Design review of the part built by this model. Coordinates are the model's own, in mm. A direction names the side the tool comes from. Give positions to 0.01 mm unless a question says otherwise; leave off trailing zeros. Loops run counter-clockwise (first coordinate to the right, second up) from the corner with the lowest first, then second, coordinate; pieces in that order, holes last. Notation, with made-up numbers: M 20,-18.5 L 62,-18.5 A26 cw 62,6.5 Z; hole C 33,41 d3. An arc over 180 degrees is marked long. Answer as CSV lines item,"result".
```python
from build123d import *

# Parameters (mm, degrees)
SKETCH1_R           = 1.5
BOSS_EXTRUDE1_DEPTH = 1.6
SKETCH2_W           = 25
SKETCH2_H           = 3
BOSS_EXTRUDE2_DEPTH = 15
SKETCH3_R           = 1.75
CUT_EXTRUDE1_DEPTH  = 25.546193697


with BuildPart() as part:
    # Sketch1 → Boss-Extrude1 (new body)
    with BuildSketch(Plane.XY):
        with BuildLine():
            Line((-9.5, -12.5), (9.5, -12.5))
            ThreePointArc((9.5, -12.5), (11.621320344, -11.621320344), (12.5, -9.5))
            Line((12.5, -9.5), (12.5, 9.5))
            ThreePointArc((12.5, 9.5), (11.621320344, 11.621320344), (9.5, 12.5))
            Line((9.5, 12.5), (-9.5, 12.5))
            ThreePointArc((-9.5, 12.5), (-11.621320344, 11.621320344), (-12.5, 9.5))
            Line((-12.5, 9.5), (-12.5, -9.5))
            ThreePointArc((-12.5, -9.5), (-11.621320344, -11.621320344), (-9.5, -12.5))
        make_face()
        with Locations((-10, 10)):
            Circle(SKETCH1_R, mode=Mode.SUBTRACT)
        with Locations(Location((10, 10, 0), (0, 0, 180))):
            Circle(SKETCH1_R, mode=Mode.SUBTRACT)
        with Locations((10, -10)):
            Circle(SKETCH1_R, mode=Mode.SUBTRACT)
        with Locations(Location((-10, -10, 0), (0, 0, 180))):
            Circle(SKETCH1_R, mode=Mode.SUBTRACT)
    extrude(amount=BOSS_EXTRUDE1_DEPTH)

    # Sketch2 → Boss-Extrude2 (add)
    with BuildSketch(Plane(origin=(0, 0, 0), x_dir=(-1, 0, 0), z_dir=(0, 0, -1))):
        with Locations((0, -3.875)):
            Rectangle(SKETCH2_W, SKETCH2_H)
    extrude(amount=BOSS_EXTRUDE2_DEPTH)

    # Sketch3 → Cut-Extrude1 (cut, through all)
    with BuildSketch(Plane(origin=(0, -2.375, 0), x_dir=(1, 0, 0), z_dir=(0, 1, 0))):
        with Locations(Location((-8, 10, 0), (0, 0, 270))):
            Circle(SKETCH3_R)
        with Locations(Location((8, 10, 0), (0, 0, 270))):
            Circle(SKETCH3_R)
    extrude(amount=-CUT_EXTRUDE1_DEPTH, mode=Mode.SUBTRACT)


solid = part.part
```
1. The part is to be moulded in two halves that separate along Z. For faces 1 (the flat face through (0, -4, -15)), 2 (the cylindrical face through (9.5, -3.9, -9.1)), 3 (the cylindrical face through (8.8, -10.9, 0.8)), say which applies: pulls with the +Z half, pulls with the -Z half, needs draft (parallel to the pull), parting line crosses it, or undercut.
Answer block:
face 1,"pulls with the -Z half"
face 2,"undercut"
face 3,"needs draft"
2. For faces 4 (the cylindrical face through (11.2, 10.9, 0.8)), 5 (the flat face through (0, 5, 0)), list the 3-axis set-ups (+Z, -Z, +X, -X, +Y, -Y) from which the entire face can be reached by the end or side of a thin tool; tool diameter is ignored.
Answer block:
face 4,"+Z, -Z"
face 5,"-Z, +X, -X, +Y"
3. We need section C-C, the plane y = 10. Write out the cut boundary in (x, z), plus the area to 3 significant figures.
Answer block:
outline,"M -12.46,0 L -11.5,0 L -11.5,1.6 L -12.46,1.6 Z; M -8.5,0 L 8.5,0 L 8.5,1.6 L -8.5,1.6 Z; M 11.5,0 L 12.46,0 L 12.46,1.6 L 11.5,1.6 Z"
area,"30.3 mm²"
4. We need section A-A, the plane x = 8. Write out the cut boundary in (y, z) (3 decimals).
Answer block:
outline,"M -12.5,0 L -5.375,0 L -5.375,-8.25 L -2.375,-8.25 L -2.375,0 L 12.5,0 L 12.5,1.6 L -12.5,1.6 Z; M -5.375,-15 L -2.375,-15 L -2.375,-11.75 L -5.375,-11.75 Z"
5. To check wall thickness, follow L1, parallel to X at y = -3.3, z = -10; L2, parallel to Y at x = 10, z = 1.2; L3, parallel to Z at x = 8, y = 11.25. State the ranges of each line that lie inside material, in increasing order. Write a range as [from, to].
Answer block:
L1,"[-12.5, -9.75], [-6.25, 6.25], [9.75, 12.5]"
L2,"[-12.46, -11.5], [-8.5, 8.5], [11.5, 12.46]"
L3,"[0, 1.6]"
6. We need section B-B, the plane z = -10. Write out the cut boundary in (x, y) (3 decimals).
Answer block:
outline,"M -12.5,-5.375 L -9.75,-5.375 L -9.75,-2.375 L -12.5,-2.375 Z; M -6.25,-5.375 L 6.25,-5.375 L 6.25,-2.375 L -6.25,-2.375 Z; M 9.75,-5.375 L 12.5,-5.375 L 12.5,-2.375 L 9.75,-2.375 Z"
7. For P1, Ø2.5, axis at x = -10, y = -10, coming from the -Z side; P2, Ø1, axis at x = 1, y = -8.5, coming from the -Z side, all flat-tipped, find the tip position at first contact; note any pin that passes through.
Answer block:
P1,"through"
P2,"z = 0"
8. We need section D-D, the plane x = -3. Write out the cut boundary in (y, z) (3 decimals).
Answer block:
outline,"M -12.5,0 L -5.375,0 L -5.375,-15 L -2.375,-15 L -2.375,0 L 12.5,0 L 12.5,1.6 L -12.5,1.6 Z"
